Model file for the job. Use its own axes, mm. Give positions to 0.01 mm unless a question says otherwise; leave off trailing zeros. Order: outer loops, then holes, each group sorted by start corner. A loop starts at its lowest first (then second) coordinate and runs counter-clockwise, first axis right, second up. Notation, with made-up numbers: M -32.75,21 L -12.75,21 A19 ccw -12.75,49 Z; hole C 79,-36 d10. An arc over 180 degrees is marked long. Return JSON: item names as keys, results as strings. Group by question number.
1. Slice it at A-A on y = -5. List the corners of the cut face in (x, z), then the cut area to 3 significant figures.
2. Pin check, flat tip, straight feed: pin 1 (4.5 mm diameter, centred on x = 110.54, y = -12.34, fed in from -Z). Stop position of the tip, or through.
3. Slice it at B-B on z = 7.5. List the corners of the cut face in (x, y).
4. Two-plate mould, pull along Y, no slides. Class faces 1 (the face through (62.286, -12.229, 24.112)), 2 (the face through (-8.814, -23.789, 10.208)), 3 (the face through (-14, -25.041, 13)), 4 (the face through (-10, -12, 2.54)): released by +Y, released by -Y, zero draft, split by the parting line, or undercut.
5. Slice it at C-C on x = 105. List the corners of the cut face in (y, z).
6. Wall check: probe 1 along Z at (x, y) = (-3, -16.75); probe 2 along Y at (x, z) = (75, 5.5); probe 3 along Z at (x, y) = (-59, -2). Give the ranges that are in metal, low to high. Write a range as [from, to].
from build123d import *

# Parameters (mm, degrees)
F0_W     = 279.4
F0_H     = 25.4
F1_DEPTH = 25.4
F2_W     = 20.32
F2_H     = 20.32
F3_DEPTH = 279.4
F6_D     = 5.1054
F7_D     = 5.1054


with BuildPart() as f1:
    # F0 (on Top) → F1 (new body)
    with BuildSketch(Plane.XY):
        with Locations((-11.921439, -12.341175)):
            Rectangle(F0_W, F0_H)
    extrude(amount=F1_DEPTH)

    # F2 (on face) → F3 (cut)
    with BuildSketch(Plane.YZ.offset(127.778561)):
        with Locations((-12.341175, 12.7)):
            Rectangle(F2_W, F2_H)
    extrude(amount=-F3_DEPTH, mode=Mode.SUBTRACT)

    # F6 (through all)
    with Locations(Plane(origin=(0, 0.358825, 0), x_dir=(-1, 0, 0), z_dir=(0, 1, 0))):
        with Locations((8.260708, 12.7), (135.260708, 12.7), (-93.339292, 12.7), (109.860708, 12.7), (-17.139292, 12.7), (-67.939292, 12.7), (33.660708, 12.7), (-118.739292, 12.7), (-42.539292, 12.7), (59.060708, 12.7), (84.460708, 12.7)):
            Hole(F6_D / 2)

    # F7 (through all)
    with Locations(Plane.XY.offset(25.4)):
        with Locations((34.336239, -12.341175), (-92.663761, -12.341175), (-16.463761, -12.341175), (-41.863761, -12.341175), (8.936239, -12.341175), (59.736239, -12.341175), (-67.263761, -12.341175), (-143.463761, -12.341175), (-118.063761, -12.341175), (85.136239, -12.341175), (110.536239, -12.341175)):
            Hole(F7_D / 2)


solid = f1.part
Result:
{
 "1": {"outline": "M -151.62,0 L 127.78,0 L 127.78,2.54 L -151.62,2.54 Z; M -151.62,22.86 L 127.78,22.86 L 127.78,25.4 L -151.62,25.4 Z", "area": "1,420 mm2"},
 "2": {"pin 1": "passes through"},
 "3": {"outline": "M -151.62,-25.04 L 127.78,-25.04 L 127.78,-22.5 L -151.62,-22.5 Z; M -151.62,-2.18 L 127.78,-2.18 L 127.78,0.36 L -151.62,0.36 Z"},
 "4": {"face 1": "undercut", "face 2": "zero draft", "face 3": "released by -Y", "face 4": "undercut"},
 "5": {"outline": "M -25.04,0 L 0.36,0 L 0.36,25.4 L -25.04,25.4 Z; hole M -22.5,2.54 L -2.18,2.54 L -2.18,22.86 L -22.5,22.86 Z"},
 "6": {"probe 1": "z = [0, 2.54], [22.86, 25.4]", "probe 2": "y = [-25.04, -22.5], [-2.18, 0.36]", "probe 3": "z = [0, 10.15], [15.25, 25.4]"}
}
